Geometry: final body of the model. Coordinates: model frame, mm. Face numbers are marked on the shaded views. A direction names the side the tool comes from. Round coordinates to 2 decimals unless told otherwise and drop trailing zeros. Write each loop counter-clockwise with the first axis right and the second up, starting at its lowest first coordinate (ties: lowest second). Pieces come first, ordered by that corner, then holes. Notation, with made-up numbers: M 24.5,-25.5 L 29.5,-25.5 A16 cw 29.5,-7.5 Z; hole C -38,51.25 d2. An arc over 180 degrees is marked long. Use one line per item in the form item = value. Start each with the question number.
Item 1: Pin query (flat end, axial travel): pin 1 Ø2 at (x, y) = (0.5, 17.5) entering from +Z; pin 2 Ø1 at (y, z) = (9.5, -3.5) entering from +X; pin 3 Ø5 at (x, y) = (-3, 13) entering from -Z; pin 4 Ø2 at (x, y) = (-2.5, 18) entering from +Z. Return the tip coordinate at first contact, or that it passes through.
Item 2: Section query A-A (z = 0). Return loops of the section in (x, y).
Item 3: Section query B-B (x = 0). Return loops of the section in (y, z), and give its area (3 significant figures).
Item 4: Section query C-C (y = 19.25). Return loops of the section in (x, z), and give its area (3 significant figures).
Item 5: Section query D-D (y = 1.75). Return loops of the section in (x, z).
Item 6: Reachability of the marked faces 1 and 2 from +Z, -Z, +X, -X, +Y, -Y: full face, straight path, thin tool, end or side. Return the list, or none.
Item 7: Ray query, probe 1 along X at (y, z) = (15.75, 0); probe 2 along Y at (x, z) = (-2.5, 1.5); probe 3 along Z at (x, y) = (-0.75, 14). Return the intervals inside material, ascending.
from build123d import *

# Parameters (mm, degrees)
SKETCH1_R           = 5
BOSS_EXTRUDE1_DEPTH = 4
SKETCH2_R           = 1.9
BOSS_EXTRUDE2_DEPTH = 17
CHAMFER1_SIZE       = 1.5
CHAMFER1_SIZE2      = 1.258649447


with BuildPart() as part:
    # Sketch1 → Boss-Extrude1 (new body)
    with BuildSketch(Plane(origin=(0, 0, 0), x_dir=(1, 0, 0), z_dir=(0, 1, 0))):
        with Locations(Location((0, 0, 0), (0, 0, 270))):
            Circle(SKETCH1_R)
    extrude(amount=BOSS_EXTRUDE1_DEPTH)

    # Sketch2 → Boss-Extrude2 (add)
    with BuildSketch(Plane(origin=(0, 4, 0), x_dir=(1, 0, 0), z_dir=(0, 1, 0))):
        with Locations(Location((0, 0, 0), (0, 0, 270))):
            Circle(SKETCH2_R)
    extrude(amount=BOSS_EXTRUDE2_DEPTH)

    # Chamfer1
    chamfer1_edges = [part.edges().sort_by_distance(p)[0] for p in [
        (0, 0, -5),
    ]]
    chamfer1_side = [part.faces().sort_by_distance(p)[0] for p in [
        (0, 0, 0),
    ]]
    chamfer(chamfer1_edges, length=CHAMFER1_SIZE, length2=CHAMFER1_SIZE2, reference=chamfer1_side[0])


solid = part.part
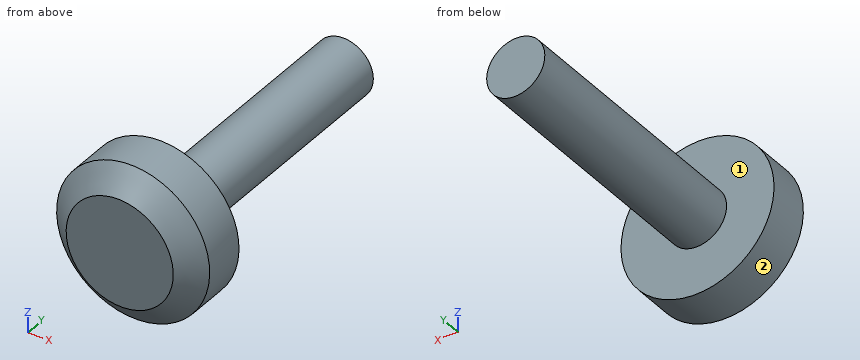
Working result:
q1.pin_1 = 1.9
q1.pin_2 = through
q1.pin_3 = -1.83
q1.pin_4 = 1.17
q2.outline = M -5,1.26 L -3.5,0 L 3.5,0 L 5,1.26 L 5,4 L 1.9,4 L 1.9,21 L -1.9,21 L -1.9,4 L -5,4 Z
q3.outline = M 0,-3.5 L 1.26,-5 L 4,-5 L 4,-1.9 L 21,-1.9 L 21,1.9 L 4,1.9 L 4,5 L 1.26,5 L 0,3.5 Z
q3.area = 103 mm²
q4.outline = C 0,0 d3.8
q4.area = 11.3 mm²
q5.outline = C 0,0 d10
q6.face_1 = +Y
q6.face_2 = +Y, -Y
q7.probe_1 = -1.9 to 1.9
q7.probe_2 = 0 to 4
q7.probe_3 = -1.75 to 1.75
